```python
from build123d import *

# Parameters (mm, degrees)
F0_W     = 101.6
F0_H     = 101.6
F1_DEPTH = 101.6
F2_W     = 101.6
F2_H     = 101.6
F3_DEPTH = 101.6
F5_DEPTH = 101.6
F6_R     = 5.08


with BuildPart() as f1:
    # F0 (on Top) → F1 (new body)
    with BuildSketch(Plane.XY):
        Rectangle(F0_W, F0_H)
    extrude(amount=F1_DEPTH)

    # F2 (on face) → F3 (join)
    with BuildSketch(Plane.XY.offset(101.6)):
        Rectangle(F2_W, F2_H)
    extrude(amount=F3_DEPTH)

    # F4 (on face) → F5 (cut)
    with BuildSketch(Plane(origin=(0, 50.8, 0), x_dir=(-1, 0, 0), z_dir=(0, 1, 0))):
        Polygon((-50.8, 101.6), (0, 203.2), (-50.8, 203.2), align=None)
        Polygon((50.8, 203.2), (0, 203.2), (50.8, 101.6), align=None)
    extrude(amount=-F5_DEPTH, mode=Mode.SUBTRACT)

    # F6
    f6_edges = [f1.edges().sort_by_distance(p)[0] for p in [
        (25.4, 50.8, 152.4),
        (50.8, 0, 101.6),
        (50.8, 50.8, 50.8),
        (0, 0, 203.2),
        (-50.8, 0, 101.6),
        (-50.8, 50.8, 50.8),
        (-50.8, 0, 0),
        (0, 50.8, 0),
        (-50.8, -50.8, 50.8),
        (50.8, -50.8, 50.8),
        (-25.4, -50.8, 152.4),
        (-25.4, 50.8, 152.4),
        (0, -50.8, 0),
        (50.8, 0, 0),
        (25.4, -50.8, 152.4),
    ]]
    fillet(f6_edges, radius=F6_R)


solid = f1.part
```
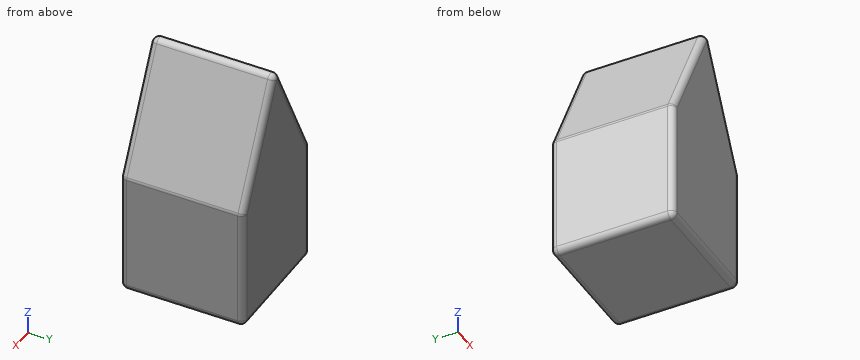
The model under review builds one solid part; all positions refer to its coordinate system, in mm. Round coordinates to 2 decimals unless told otherwise and drop trailing zeros. Write each loop counter-clockwise with the first axis right and the second up, starting at its lowest first coordinate (ties: lowest second). Pieces come first, ordered by that corner, then holes.
(1) Wall thickness on L1, parallel to X at y = 24, z = 142; L2, parallel to Z at x = -23.5, y = 28; L3, parallel to X at y = 34.5, z = 115: over which ranges is each line inside the solid? List them lowest first.
(2) Insertion check: pin 1 (6 mm diameter, centred on y = -24.5, z = 139.5, fed in from -X); pin 2 (12 mm diameter, centred on y = -17.5, z = 144.5, fed in from -X). Each pin has a flat end and moves straight along its axis. Give the tip position at first contact, or say it passes through.
(3) We need section A-A on y = 35.5. Give the boundary of the cut face in (x, z).
Findings below:
1. L1: x = -30.6 to 30.6
1. L2: z = 0 to 156.2
1. L3: x = -44.1 to 44.1
2. pin 1: stops at x = -33.35
2. pin 2: stops at x = -32.35
3. outline: (-50.8, 5.08) arc R5.08 ccw to (-45.72, 0) - (45.72, 0) arc R5.08 ccw to (50.8, 5.08) - (50.8, 100.4) arc R5.08 ccw to (50.26, 102.67) - (4.54, 194.11) arc R5.08 ccw to (-4.54, 194.11) - (-50.26, 102.67) arc R5.08 ccw to (-50.8, 100.4) - close
